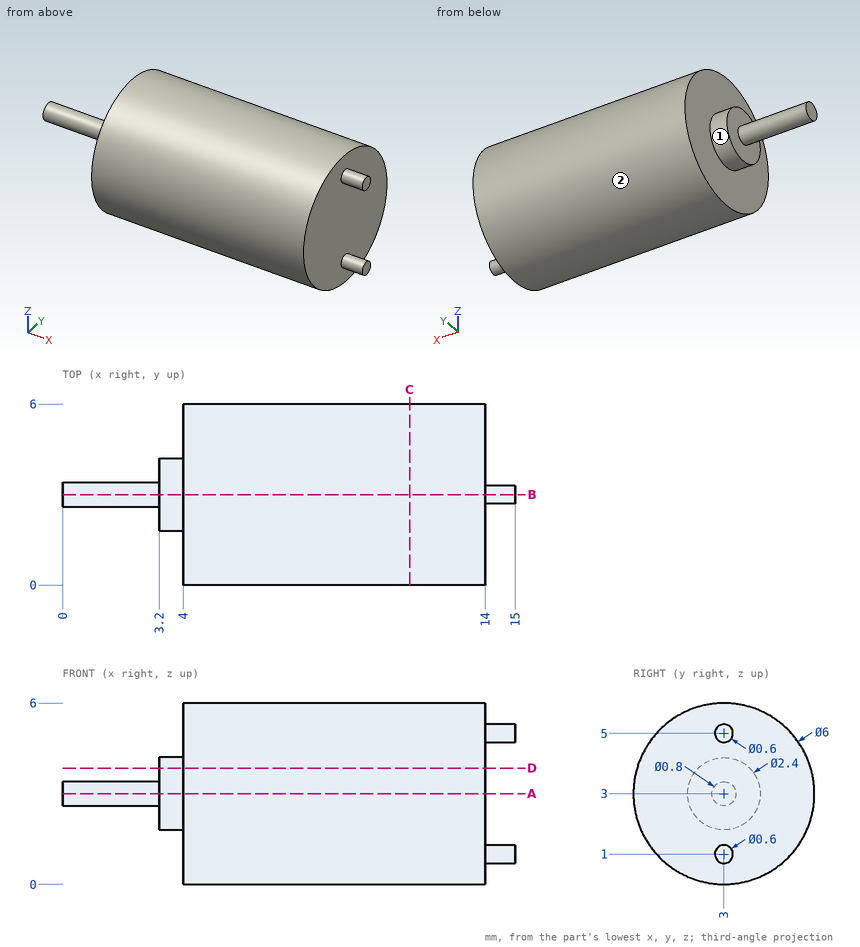
Here's the drawing with two shaded views (mm, measured from the low corner). I have some questions. A direction names the side the tool comes from. Round coordinates to 2 decimals unless told otherwise and drop trailing zeros. Loops run counter-clockwise (first coordinate to the right, second up) from the corner with the lowest first, then second, coordinate; pieces in that order, holes last. Notation, with made-up numbers: M 11,13 L 51,13 A22 cw 51,32 Z; hole C -6,-9.5 d5. An arc over 180 degrees is marked long. Answer as a JSON object with one key per item and string values. Group by question number.
Q1. Imagine slicing it at A-A, the plane z = 3. Please give me the cut outline in (x, y).
Q2. Imagine slicing it at B-B, the plane y = 3. Please give me the cut outline in (x, z), then the cut area to 3 significant figures.
Q3. Will these pins go through, and if not, where does the flat tip stop? pin 1 (1.9 mm diameter, centred on y = 3.5, z = 3.5, fed in from -X); pin 2 (3 mm diameter, centred on x = 3.5, z = 1.5, fed in from +Y).
Q4. Please list where these lines run through material, in increasing order: L1, parallel to X at y = 3.6, z = 2.3; L2, parallel to X at y = 1.3, z = 3.35; L3, parallel to Y at x = 9.5, z = 5.55.
Q5. On a 3-axis mill with a long thin cutter (end or side, diameter ignored), from which of +Z, -Z, +X, -X, +Y, -Y can I reach the whole of each face in a straight line? I mean the marked faces 1 and 2. Say none if no direction works.
Q6. Imagine slicing it at C-C, the plane x = 11.5. Please give me the cut outline in (y, z), then the cut area to 3 significant figures.
Q7. Imagine slicing it at D-D, the plane z = 3.85. Please give me the cut outline in (x, y), then the cut area to 3 significant figures.
Findings:
{
 "1": {"outline": "M 0,2.6 L 3.2,2.6 L 3.2,1.8 L 4,1.8 L 4,0 L 14,0 L 14,6 L 4,6 L 4,4.2 L 3.2,4.2 L 3.2,3.4 L 0,3.4 Z"},
 "2": {"outline": "M 0,2.6 L 3.2,2.6 L 3.2,1.8 L 4,1.8 L 4,0 L 14,0 L 14,0.7 L 15,0.7 L 15,1.3 L 14,1.3 L 14,4.7 L 15,4.7 L 15,5.3 L 14,5.3 L 14,6 L 4,6 L 4,4.2 L 3.2,4.2 L 3.2,3.4 L 0,3.4 Z", "area": "65.7 mm2"},
 "3": {"pin 1": "stops at x = 0", "pin 2": "stops at y = 6"},
 "4": {"L1": "x = 3.2 to 14", "L2": "x = 4 to 14", "L3": "y = 1.42 to 4.58"},
 "5": {"face 1": "-X", "face 2": "+X, -X"},
 "6": {"outline": "C 3,3 d6", "area": "28.3 mm2"},
 "7": {"outline": "M 3.2,2.15 L 4,2.15 L 4,0.12 L 14,0.12 L 14,5.88 L 4,5.88 L 4,3.85 L 3.2,3.85 Z", "area": "58.9 mm2"}
}
